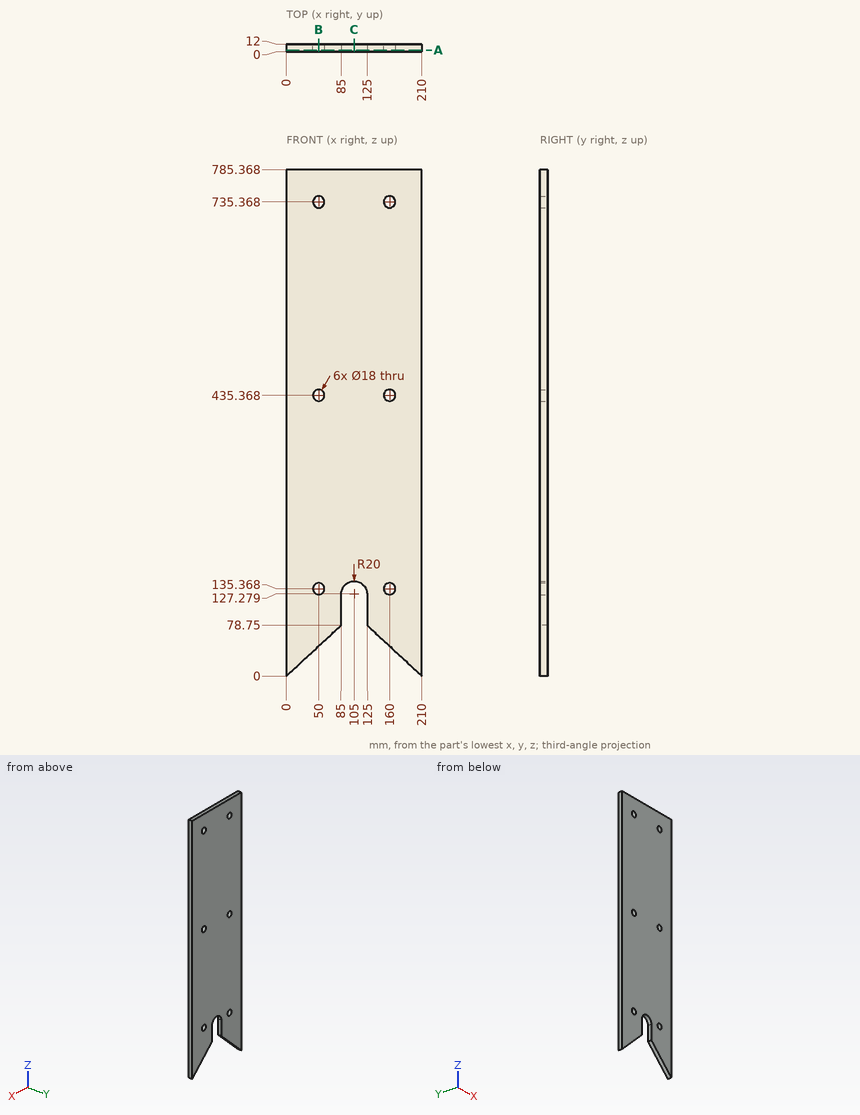
Geometry check sheet. Reference: drawing and pictorial views, mm from the part's lowest x, y, z. Coordinates: 2 decimals unless noted, no trailing zeros. Order: outer loops, then holes, each group sorted by start corner. A loop starts at its lowest first (then second) coordinate and runs counter-clockwise, first axis right, second up. Notation, with made-up numbers: (51.25, 76) - (72.25, 76) arc R31 ccw to (72.25, 109) - close; hole circle Ø7 at (77, 49). An arc over 180 degrees is marked (long way). Answer in a Markdown table with one row per item. Add a question column.
1) Material ranges on line 1 along Z through (x, y) = (160, 6.25) (1 decimal); line 2 along X through (y, z) = (2, 433); line 3 along Z through (x, y) = (162, 8.25) (1 decimal), recorded low to high. Write a range as [from, to].
2) Gauge pin test, flat ends, axial feed: P1, Ø11, axis at x = 50, z = 435.37, coming from the -Y side; P2, Ø4, axis at x = 85.5, y = 10, coming from the -Z side; P3, Ø5, axis at x = 185, y = 1.5, coming from the -Z side (1 decimal). Record the tip position at first contact, or that the pin passes through.
3) Cross-section at C-C, the plane x = 105. Record the cut outline in (y, z), then the cut area to 3 significant figures.
4) Cross-section at B-B, the plane x = 50. Record the cut outline in (y, z), then the cut area to 3 significant figures.
5) Cross-section at A-A, the plane y = 2.5. Record the cut outline in (x, z).
Check result:
| question | item | result |
|---|---|---|
| 1 | line 1 | z = [46.3, 126.4], [144.4, 426.4], [444.4, 726.4], [744.4, 785.4] |
| 1 | line 2 | x = [0, 41.32], [58.68, 151.32], [168.68, 210] |
| 1 | line 3 | z = [44.5, 126.6], [144.1, 426.6], [444.1, 726.6], [744.1, 785.4] |
| 2 | P1 | passes through |
| 2 | P2 | stops at z = 77.36 |
| 2 | P3 | stops at z = 20.8 |
| 3 | outline | (0, 147.28) - (12, 147.28) - (12, 785.37) - (0, 785.37) - close |
| 3 | area | 7,660 mm² |
| 4 | outline | (0, 46.32) - (12, 46.32) - (12, 126.37) - (0, 126.37) - close; (0, 144.37) - (12, 144.37) - (12, 426.37) - (0, 426.37) - close; (0, 444.37) - (12, 444.37) - (12, 726.37) - (0, 726.37) - close; (0, 744.37) - (12, 744.37) - (12, 785.37) - (0, 785.37) - close |
| 4 | area | 8,220 mm² |
| 5 | outline | (0, 0) - (85, 78.75) - (85, 127.28) arc R20 cw to (125, 127.28) - (125, 78.75) - (210, 0) - (210, 785.37) - (0, 785.37) - close; hole circle Ø18 at (50, 135.37); hole circle Ø18 at (50, 435.37); hole circle Ø18 at (50, 735.37); hole circle Ø18 at (160, 135.37); hole circle Ø18 at (160, 435.37); hole circle Ø18 at (160, 735.37) |
